```python
from build123d import *

# Parameters (mm, degrees)
SKETCH_1_R                        = 4
EXTRUDE_1_DEPTH                   = 10
CUT_EXTRUDE_1_DEPTH               = 62.489836559
CUT_EXTRUDE_1_DEPTH_BACK          = 62.489836559
HOLE_WIZARD_6_5_6_5_1_D           = 6.5
HOLE_WIZARD_6_5_6_5_1_DEPTH       = 13
HOLE_WIZARD_6_5_6_5_1_CSINK_D     = 13
HOLE_WIZARD_6_5_6_5_1_CSINK_ANGLE = 90
HOLE_WIZARD_6_5_6_5_1_TIP         = 1.952797012
FILLET_1_R                        = 5


# Read off the part's stored shape, not the designer's step: M5 螺纹孔1
with BuildPart() as part:
    # 草图1 → 凸台-拉伸1 (new, symmetric)
    with BuildSketch(Plane.XY):
        with BuildLine():
            Line((0, 0), (51, 0))
            ThreePointArc((51, 0), (57.363961031, 15.363961031), (42, 9))
            Line((42, 9), (0, 9))
            Line((0, 9), (0, 0))
        make_face()
        with Locations((51, 9)):
            Circle(SKETCH_1_R, mode=Mode.SUBTRACT)
    extrude(amount=EXTRUDE_1_DEPTH, both=True)

    # 草图2 → 切除-拉伸1 (cut, two sides: drawn at the far end of the back side and taken through both)
    with BuildSketch(Plane(origin=(0, 9, 0), x_dir=(1, 0, 0), z_dir=(0, 1, 0)).offset(-CUT_EXTRUDE_1_DEPTH_BACK)):
        Polygon((193.693168769, 5), (60, 5), (38, 5), (38, 10), (38, 143.693168769), (215.856075393, 343.349548449), (371.549244162, 204.65637968), align=None)
    extrude(amount=CUT_EXTRUDE_1_DEPTH + CUT_EXTRUDE_1_DEPTH_BACK, mode=Mode.SUBTRACT)

    # Ø6.5 (6.5) 直径孔1
    with Locations(Plane(origin=(0, 9, 0), x_dir=(1, 0, 0), z_dir=(0, 1, 0))):
        with Locations((11, 0), (27, 0)):
            CounterSinkHole(HOLE_WIZARD_6_5_6_5_1_D / 2, HOLE_WIZARD_6_5_6_5_1_CSINK_D / 2, depth=HOLE_WIZARD_6_5_6_5_1_DEPTH, counter_sink_angle=HOLE_WIZARD_6_5_6_5_1_CSINK_ANGLE)
            with Locations((0, 0, -(HOLE_WIZARD_6_5_6_5_1_DEPTH + HOLE_WIZARD_6_5_6_5_1_TIP / 2))):  # 118° drill point
                Cone(0, HOLE_WIZARD_6_5_6_5_1_D / 2, HOLE_WIZARD_6_5_6_5_1_TIP, mode=Mode.SUBTRACT)

    # M5 螺纹孔1 outline → M5 螺纹孔1 (revolve, cut)
    with BuildSketch(Plane(origin=(51, 0, 2), x_dir=(1, 0, 0), z_dir=(0, 0, 1))):
        Polygon((2.52510553, 18.00010553), (0, 18.00010553), (0, 12.404132041), (2.1, 12.404132041), (2.1, 17.575), align=None)
    revolve(axis=Axis((51, 0, 2), (0, 1, 0)), mode=Mode.SUBTRACT)

    # 圆角1
    fillet_1_edges = [part.edges().sort_by_distance(p)[0] for p in [
        (0, 4.5, 10),
        (0, 4.5, -10),
    ]]
    fillet(fillet_1_edges, radius=FILLET_1_R)


solid = part.part
```
Model file for the job. Use its own axes, mm. A direction names the side the tool comes from. Give positions to 0.01 mm unless a question says otherwise; leave off trailing zeros. Write each loop counter-clockwise with the first axis right and the second up, starting at its lowest first coordinate (ties: lowest second). Pieces come first, ordered by that corner, then holes. Notation, with made-up numbers: (75.25, 76.25) -> (109.25, 76.25) arc R33 cw to (109.25, 110.25) -> close; hole circle Ø8 at (-39.75, -9.75). An arc over 180 degrees is marked (long way). Use CSV: the item, a comma, the result in double quotes. Start each with the question number.
1) Cut at A-A on y = 7. List the corners of the cut face in (x, z).
2) Cut at D-D on x = 54. List the corners of the cut face in (y, z).
3) Tool access for faces 1 (the flat face through (38, 4, -8)), 2 (the cylindrical face through (48.9, 15.03, 1.91)), 3 (the flat face through (21, 9, 5)), 4 (the cylindrical face through (1, 4, -8)), 5 (the flat face through (0, 5, 0)): list every direction of +Z, -Z, +X, -X, +Y, -Y with a clear straight run to the whole face (end or side of a thin tool).
4) Cut at C-C on z = 9. List the corners of the cut face in (x, y), plus the area to 3 significant figures.
5) Pin check, flat tips, straight feed: P1, Ø2.5, axis at y = 3, z = -6.5, coming from the +X side; P2, Ø10, axis at y = 2, z = 5, coming from the +X side; P3, Ø7.5, axis at x = 11, z = 0, coming from the +Y side. Stop position of each tip, or through.
6) Drill centre lines: L1, parallel to Z at x = 27, y = 3.85; L2, parallel to X at y = 10.5, z = 4; L3, parallel to X at y = 14, z = 2. Where is each one in solid material? Low to high.
7) Cut at B-B on x = 11. List the corners of the cut face in (y, z), plus the area to 3 significant figures.
8) Two-plate mould, pull along X, no slides. Class faces 6 (the cylindrical face through (1, 4, 8)), 7 (the cylindrical face through (14.247, 2.835, -0.143)), 8 (the flat face through (46, 7, -5)): released by +X, released by -X, zero draft, split by the parting line, or undercut.
Final values:
1,outline,"(0, -5) arc R5 ccw to (5, -10) -> (38, -10) -> (38, -5) -> (47.54, -5) -> (47.54, 10) -> (5, 10) arc R5 ccw to (0, 5) -> close; (54.46, -5) -> (59.77, -5) -> (59.77, 10) -> (54.46, 10) -> close; hole circle Ø9 at (11, 0); hole circle Ø9 at (27, 0)"
2,outline,"(0.51, -5) -> (6.35, -5) -> (6.35, 10) -> (0.51, 10) -> close; (11.65, -5) -> (17.49, -5) -> (17.49, 10) -> (11.65, 10) -> close"
3,face 1,"-Z, +X, +Y, -Y"
3,face 2,"+Y"
3,face 3,"+Z, -Z, -X, +Y"
3,face 4,"-Z, -X, +Y, -Y"
3,face 5,"+Z, -Z, -X, +Y, -Y"
4,outline,"(2, 0) -> (51, 0) arc R9 ccw (long way) to (42, 9) -> (2, 9) -> close; hole circle Ø8 at (51, 9)"
4,area,"582 mm2"
5,P1,"stops at x = 38"
5,P2,"stops at x = 59.77"
5,P3,"stops at y = 6.25"
6,L1,"z = -10 to -3.25, 3.25 to 10"
6,L2,"x = 42.13 to 47.29, 54.71 to 59.87"
6,L3,"x = 43.52 to 48.9, 53.1 to 58.48"
7,outline,"(0, -10) -> (9, -10) -> (9, -6.5) -> (5.75, -3.25) -> (0, -3.25) -> close; (0, 3.25) -> (5.75, 3.25) -> (9, 6.5) -> (9, 10) -> (0, 10) -> close"
7,area,"111 mm2"
8,face 6,"released by -X"
8,face 7,"undercut"
8,face 8,"zero draft"
